Geometry check sheet. Reference: the model listing, model coordinates, mm. A direction names the side the tool comes from. Round coordinates to 2 decimals unless told otherwise and drop trailing zeros. Write each loop counter-clockwise with the first axis right and the second up, starting at its lowest first coordinate (ties: lowest second). Pieces come first, ordered by that corner, then holes. Notation, with made-up numbers: (19.5, -22) -> (75.5, -22) arc R24 cw to (75.5, -11) -> close; hole circle Ø5 at (21, -27). An arc over 180 degrees is marked (long way). Put each result on its own line as item: value. Start each with the question number.
from build123d import *

# Parameters (mm, degrees)
F0_W     = 38.1
F0_H     = 76.2
F1_DEPTH = 1.27
F2_W     = 1.27
F2_H     = 1.27
F2_W_2   = 35.56
F2_H_2   = 73.66
F3_DEPTH = 101.6
F4_W     = 38.1
F4_H     = 76.2
F5_DEPTH = 1.27
F7_R     = 3.75
F7_R_2   = 4.25
F7_R_3   = 5
F7_R_4   = 5.75
F7_R_5   = 6.25
F8_DEPTH = 25.4


with BuildPart() as f1:
    # F0 (on Top) → F1 (new body)
    with BuildSketch(Plane.XY):
        Rectangle(F0_W, F0_H)
    extrude(amount=F1_DEPTH)

    # F2 (on face) → F3 (join)
    with BuildSketch(Plane.XY.offset(1.27)):
        with Locations((-18.415, 37.465)):
            Rectangle(F2_W, F2_H)
        with Locations((0, 37.465)):
            Rectangle(F2_W_2, F2_H)
        with Locations((-18.415, 0)):
            Rectangle(F2_W, F2_H_2)
        with Locations((18.415, 37.465)):
            Rectangle(F2_W, F2_H)
        with Locations((-18.415, -37.465)):
            Rectangle(F2_W, F2_H)
        with Locations((0, -37.465)):
            Rectangle(F2_W_2, F2_H)
        with Locations((18.415, 0)):
            Rectangle(F2_W, F2_H_2)
        with Locations((18.415, -37.465)):
            Rectangle(F2_W, F2_H)
    extrude(amount=F3_DEPTH)

    # F4 (on face) → F5 (join)
    with BuildSketch(Plane.XY.offset(102.87)):
        Rectangle(F4_W, F4_H)
    extrude(amount=F5_DEPTH)

    # F7 (on face) → F8 (cut)
    with BuildSketch(Plane.XY.offset(104.14)):
        with Locations((-8.89, 30.48)):
            Circle(F7_R)
        with Locations((8.89, 30.48)):
            Circle(F7_R)
        with Locations((-8.89, 17.78)):
            Circle(F7_R_2)
        with Locations((8.89, 17.78)):
            Circle(F7_R_2)
        with Locations((8.89, 3.81)):
            Circle(F7_R_3)
        with Locations((-8.89, 3.81)):
            Circle(F7_R_3)
        with Locations((-8.89, -11.43)):
            Circle(F7_R_4)
        with Locations((8.89, -11.43)):
            Circle(F7_R_4)
        with Locations((8.89, -27.94)):
            Circle(F7_R_5)
        with Locations((-8.89, -27.94)):
            Circle(F7_R_5)
    extrude(amount=-F8_DEPTH, mode=Mode.SUBTRACT)


solid = f1.part
(1) Material ranges on L1, parallel to Y at x = 8.89, z = 103.5; L2, parallel to X at y = -2.5, z = 36; L3, parallel to Z at x = -6, y = -3.5, recorded low to high. Write a range as from..to.
(2) Sectioned sample at D-D (y = 17.78). Record the cut outline in (x, z).
(3) Go/stop test with a flat-tipped pin: pin 1 Ø6 at (x, y) = (-8.89, 30.48) entering from +Z. Record where the tip stops, or that it passes through.
(4) Set-up check for faces 5 (the flat face through (0, 1, 1.27)), 6 (the flat face through (0, 38.1, 51)), 7 (the cylindrical face through (11.543, -16.531, 103.514)): record each of +Z, -Z, +X, -X, +Y, -Y from which the full face is reachable in a straight line by a thin tool's end or side.
(5) Sectioned sample at A-A (y = -27.94). Record the cut outline in (x, z).
(6) Mould release check, pull along X, two halves, no side actions. Record for faces 1 (the flat face through (-19.05, -1, 51)), 2 (the flat face through (19.05, -1, 51)), 3 (the cylindrical face through (10.85, 14.01, 103.51)), 4 (the flat face through (0, 1, 0)): +X half, -X half, draft (parallel to the pull), parting line (faces both ways), or undercut.
(7) Sectioned sample at C-C (z = 42.5). Record the cut outline in (x, y).
(8) Sectioned sample at B-B (x = -8.89). Record the cut outline in (y, z).
Found:
1. L1: -38.1..-34.19, -21.69..-17.18, -5.68..-1.19, 8.81..13.53, 22.03..26.73, 34.23..38.1
1. L2: -19.05..-17.78, 17.78..19.05
1. L3: 0..1.27, 102.87..104.14
2. outline: (-19.05, 0) -> (19.05, 0) -> (19.05, 104.14) -> (13.14, 104.14) -> (13.14, 102.87) -> (17.78, 102.87) -> (17.78, 1.27) -> (-17.78, 1.27) -> (-17.78, 102.87) -> (-13.14, 102.87) -> (-13.14, 104.14) -> (-19.05, 104.14) -> close; (-4.64, 102.87) -> (4.64, 102.87) -> (4.64, 104.14) -> (-4.64, 104.14) -> close
3. pin 1: z = 1.27
4. face 5: none
4. face 6: +Z, -Z, +X, -X, +Y
4. face 7: +Z
5. outline: (-19.05, 0) -> (19.05, 0) -> (19.05, 104.14) -> (15.14, 104.14) -> (15.14, 102.87) -> (17.78, 102.87) -> (17.78, 1.27) -> (-17.78, 1.27) -> (-17.78, 102.87) -> (-15.14, 102.87) -> (-15.14, 104.14) -> (-19.05, 104.14) -> close; (-2.64, 102.87) -> (2.64, 102.87) -> (2.64, 104.14) -> (-2.64, 104.14) -> close
6. face 1: -X half
6. face 2: +X half
6. face 3: undercut
6. face 4: draft
7. outline: (-19.05, -38.1) -> (19.05, -38.1) -> (19.05, 38.1) -> (-19.05, 38.1) -> close; hole (-17.78, -36.83) -> (17.78, -36.83) -> (17.78, 36.83) -> (-17.78, 36.83) -> close
8. outline: (-38.1, 0) -> (38.1, 0) -> (38.1, 104.14) -> (34.23, 104.14) -> (34.23, 102.87) -> (36.83, 102.87) -> (36.83, 1.27) -> (-36.83, 1.27) -> (-36.83, 102.87) -> (-34.19, 102.87) -> (-34.19, 104.14) -> (-38.1, 104.14) -> close; (-21.69, 102.87) -> (-17.18, 102.87) -> (-17.18, 104.14) -> (-21.69, 104.14) -> close; (-5.68, 102.87) -> (-1.19, 102.87) -> (-1.19, 104.14) -> (-5.68, 104.14) -> close; (8.81, 102.87) -> (13.53, 102.87) -> (13.53, 104.14) -> (8.81, 104.14) -> close; (22.03, 102.87) -> (26.73, 102.87) -> (26.73, 104.14) -> (22.03, 104.14) -> close
